```python
from build123d import *

# Parameters (mm, degrees)
F1_DEPTH = 63.5
F0_W     = 25.4
F0_H     = 19.05
F2_DEPTH = 25.4
F3_DEPTH = 7.9375
F5_R     = 8.89
F6_R     = 15.875
F7_DEPTH = 38.1
F8_R     = 4.572


with BuildPart() as f1:
    # F0 (on Front) → F1 (new body, symmetric)
    with BuildSketch(Plane.XZ):
        Polygon((-41.275, -9.525), (41.275, -9.525), (41.275, 9.525), (22.225, 9.525), (-41.275, 9.525), align=None)
    extrude(amount=F1_DEPTH, both=True)

    # F0 (on Front) → F2 (join, symmetric)
    with BuildSketch(Plane.XZ):
        with BuildLine():
            Line((22.225, 9.525), (41.275, 9.525))
            Line((41.275, 9.525), (41.275, 27.0002))
            ThreePointArc((41.275, 27.0002), (45.9246798487, 38.2255201513), (57.15, 42.8752))
            Line((57.15, 42.8752), (60.325, 42.8752))
            Line((60.325, 42.8752), (60.325, 61.9252))
            Line((60.325, 61.9252), (57.15, 61.9252))
            ThreePointArc((57.15, 61.9252), (32.4542956671, 51.6959043329), (22.225, 27.0002))
            Line((22.225, 27.0002), (22.225, 9.525))
        make_face()
        with Locations((73.025, 52.4002)):
            Rectangle(F0_W, F0_H)
    extrude(amount=F2_DEPTH, both=True)

    # F0 (on Front) → F3 (join, symmetric)
    with BuildSketch(Plane.XZ):
        with BuildLine():
            add(Edge.make_bspline(
                [(-41.275, 9.525), (-41.656780988, 42.0436710119), (0, 93.9072296023), (57.15, 61.9252)],
                knots=[0, 0, 0, 0, 111.5045361635, 111.5045361635, 111.5045361635, 111.5045361635], degree=3))
            Line((-41.275, 9.525), (22.225, 9.525))
            Line((22.225, 9.525), (22.225, 27.0002))
            ThreePointArc((22.225, 27.0002), (32.4542956671, 51.6959043329), (57.15, 61.9252))
        make_face()
    extrude(amount=F3_DEPTH, both=True)

    # F0 (on Front) → F4 (revolve)
    with BuildSketch(Plane.XZ):
        Polygon((85.725, 66.675), (85.725, 61.9252), (85.725, 42.8752), (85.725, 28.575), (111.125, 28.575), (111.125, 66.675), align=None)
    revolve(axis=Axis((85.725, 0, 47.625), (0, 0, 1)))

    # F5
    f5_edges = [f1.edges().sort_by_distance(p)[0] for p in [
        (-41.275, -63.5, 0),
        (41.275, -63.5, 0),
        (41.275, 63.5, 0),
        (-41.275, 63.5, 0),
    ]]
    fillet(f5_edges, radius=F5_R)

    # F6 (on face) → F7 (cut, through all)
    with BuildSketch(Plane.XY.offset(66.675)):
        with Locations((85.725, 0)):
            Circle(F6_R)
    extrude(amount=-F7_DEPTH, mode=Mode.SUBTRACT)

    # F8
    f8_edges = [f1.edges().sort_by_distance(p)[0] for p in [
        (69.85, 0, 66.675),
        (69.85, 0, 28.575),
        (60.325, 0, 66.675),
        (60.325, 0, 28.575),
    ]]
    fillet(f8_edges, radius=F8_R)


solid = f1.part
```
Geometry check sheet. Reference: the model listing, model coordinates, mm. A direction names the side the tool comes from. Coordinates: 2 decimals unless noted, no trailing zeros. Order: outer loops, then holes, each group sorted by start corner. A loop starts at its lowest first (then second) coordinate and runs counter-clockwise, first axis right, second up.
Item 1: Tool access check on faces 1 (the flat face through (60, 2, 42.875)), 2 (the cylindrical face through (32.73, 16.55, 51.97)), 3 (the flat face through (22.225, -17, 18)). Record the directions out of +Z, -Z, +X, -X, +Y, -Y that give a thin tool (end or side, any length) a straight path to the whole face; none if there is none.
Item 2: Section check A-A (z = -4). Enter the section's corners in (x, y) (3 decimals), plus the area to 3 significant figures.
Item 3: Mould release check, pull along X, two halves, no side actions. Record for faces 4 (the cylindrical face through (73.127, -9.66, 47.828)), 5 (the flat face through (-1, -1, -9.525)), 6 (the flat face through (41.275, -1, 4)): released by +X, released by -X, zero draft, split by the parting line, or undercut.
Item 4: Scan lines: line 1 along X through (y, z) = (25, -4) (3 decimals); line 2 along Z through (x, y) = (-2.5, -22.5) (3 decimals); line 3 along Y through (x, z) = (9, 68). Record each from-to range of solid material in increasing order.
Item 5: Depth check by flat-ended pin: pin 1 (2 mm diameter, centred on x = 57, z = 51.5, fed in from +Y); pin 2 (1.5 mm diameter, centred on x = -17.5, z = 56, fed in from +Y); pin 3 (10 mm diameter, centred on x = 81, z = 26.5, fed in from -Y). Enter the tip coordinate at first touch or a pass-through.
Item 6: Section check C-C (y = -46.5). Enter the section's corners in (x, z) (3 decimals), plus the area to 3 significant figures.
Item 7: Section check B-B (z = 31). Count the separate pieces of the cut face and the enclosed holes in it, plus the area to 3 significant figures.
Check sheet entries:
1. face 1: -Z
1. face 2: +Z, -X, +Y
1. face 3: +Z, -X, -Y
2. outline: (-41.275, -54.61) arc R8.89 ccw to (-32.385, -63.5) - (32.385, -63.5) arc R8.89 ccw to (41.275, -54.61) - (41.275, 54.61) arc R8.89 ccw to (32.385, 63.5) - (-32.385, 63.5) arc R8.89 ccw to (-41.275, 54.61) - close
2. area: 10,400 mm2
3. face 4: undercut
3. face 5: zero draft
3. face 6: released by +X
4. line 1: x = -41.275 to 41.275
4. line 2: z = -9.525 to 9.525
4. line 3: y = -7.94 to 7.94
5. pin 1: stops at y = 25.4
5. pin 2: stops at y = 7.94
5. pin 3: stops at y = -24.79
6. outline: (-41.275, -9.525) - (41.275, -9.525) - (41.275, 9.525) - (-41.275, 9.525) - close
6. area: 1,570 mm2
7. separate pieces: 2
7. enclosed holes: 1
7. area: 3,010 mm2
